from build123d import *

# Parameters (mm, degrees)
PAD_DEPTH = 200
FILLET_R  = 6


with BuildPart() as part:
    # Sketch → Pad (new body)
    with BuildSketch(Plane.XY):
        Polygon((0, 0), (0, 13), (8, 13), (8, 8), (58, 8), (58, 0), align=None)
    extrude(amount=PAD_DEPTH)

    # Fillet
    fillet_edges = [part.edges().sort_by_distance(p)[0] for p in [
        (58, 0, 100),
        (0, 0, 100),
        (0, 13, 100),
    ]]
    fillet(fillet_edges, radius=FILLET_R)


solid = part.part
Can you work these out from the model? Positions are in its coordinate system, mm. A direction names the side the tool comes from. Round coordinates to 2 decimals unless told otherwise and drop trailing zeros. Write each loop counter-clockwise with the first axis right and the second up, starting at its lowest first coordinate (ties: lowest second). Pieces come first, ordered by that corner, then holes. Notation, with made-up numbers: M 1.5,1.5 L 42.5,1.5 A27 cw 42.5,38.5 Z; hole C -36,-4.75 d4. An arc over 180 degrees is marked long. Use CSV: the item, a comma, the result in double quotes.
(1) On a 3-axis mill with a long thin cutter (end or side, diameter ignored), from which of +Z, -Z, +X, -X, +Y, -Y can I reach the whole of each face in a straight line? I mean faces 1 (the cylindrical face through (56.289, 1.804, 101.4)), 2 (the flat face through (33, 8, 99)). Say none if no direction works.
Check values:
face 1,"+Z, -Z, +X, -Y"
face 2,"+Z, -Z, +X, +Y"
(2) I'm going to push flat-ended pins straight in: pin 1 (12 mm diameter, centred on x = 35.5, z = 164.5, fed in from +Y); pin 2 (4 mm diameter, centred on y = 11.5, z = 80.5, fed in from +X); pin 3 (4 mm diameter, centred on y = 9.5, z = 156.5, fed in from -X). Where does each tip first touch, or does it pass through?
Check values:
pin 1,"y = 8"
pin 2,"x = 8"
pin 3,"x = 0.02"
(3) I need wall thicknesses on line 1 along Y through (x, z) = (29, 9.5); line 2 along X through (y, z) = (5.5, 40); line 3 along X through (y, z) = (5, 108.5). Which ranges of each line are inside material? Lowest first, please.
Check values:
line 1,"0 to 8"
line 2,"0.02 to 57.98"
line 3,"0.08 to 57.92"
(4) Imagine slicing it at C-C (y = 3.5). Write out the boundary of the cut face in (x, z).
Check values:
outline,"M 0.55,0 L 57.45,0 L 57.45,200 L 0.55,200 Z"
(5) Imagine slicing it at B-B (x = 30). Write out the boundary of the cut face in (y, z), plus the area to 3 significant figures.
Check values:
outline,"M 0,0 L 8,0 L 8,200 L 0,200 Z"
area,"1,600 mm^2"
(6) Imagine slicing it at A-A (z = 16). Write out the boundary of the cut face in (x, y).
Check values:
outline,"M 0,6 A6 ccw 6,0 L 52,0 A6 ccw 58,6 L 58,8 L 8,8 L 8,13 L 6,13 A6 ccw 0,7 Z"
